Geometry: see drawing. Coordinates: mm, zero at the bounding-box minimum. A direction names the side the tool comes from. Coordinates: 2 decimals unless noted, no trailing zeros. Order: outer loops, then holes, each group sorted by start corner. A loop starts at its lowest first (then second) coordinate and runs counter-clockwise, first axis right, second up.
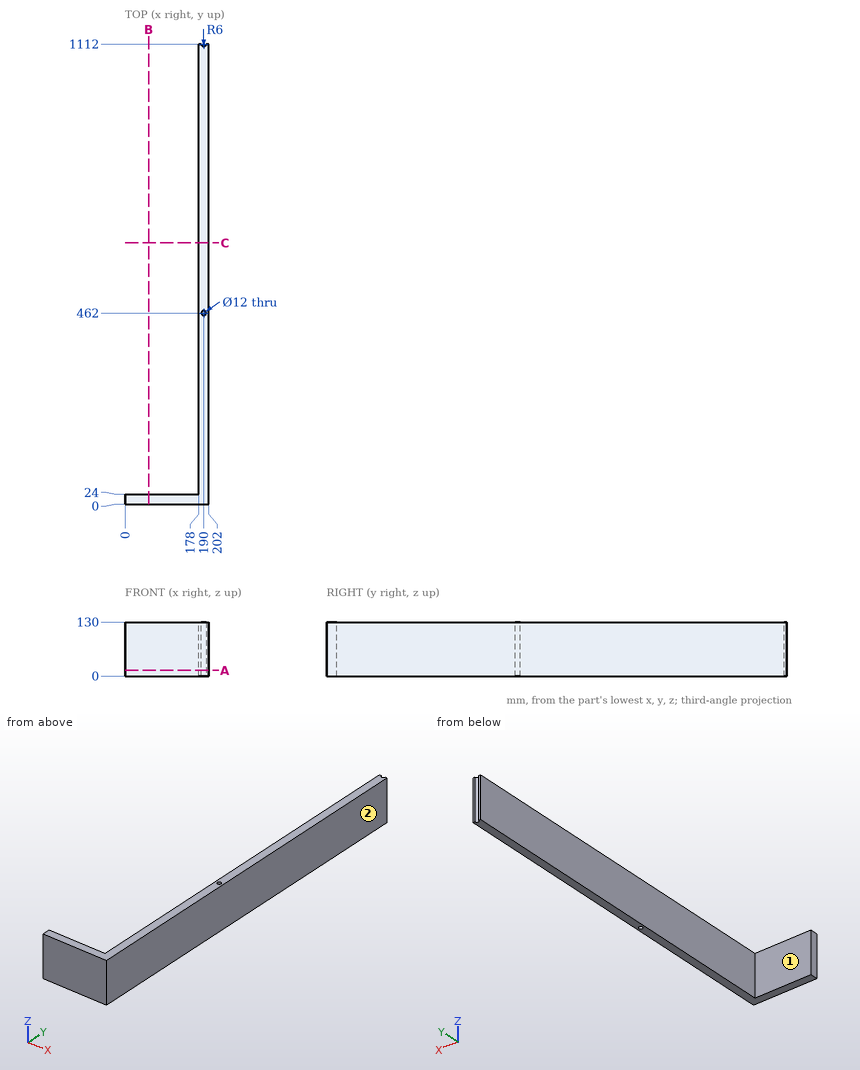
Item 1: Cut plane A-A on z = 13.5. Return loops of the section in (x, y), then the cut area to 3 significant figures.
Response values:
outline: (0, 0) - (202, 0) - (202, 1112) - (196, 1112) arc R6 cw to (184, 1112) - (178, 1112) - (178, 24) - (0, 24) - close; hole circle Ø12 at (190, 462)
area: 30,800 mm2
Item 2: Pin query (flat end, axial travel): pin 1 Ø2 at (x, z) = (142, 88) entering from +Y; pin 2 Ø8 at (y, z) = (142, 54.5) entering from -X; pin 3 Ø3 at (x, y) = (180, 131.5) entering from -Z. Return the tip coordinate at first contact, or that it passes through.
Response values:
pin 1: stops at y = 24
pin 2: stops at x = 178
pin 3: stops at z = 0
Item 3: Access query for the marked faces 1 and 2. Directions: +Z, -Z, +X, -X, +Y, -Y. A direction counts if a zero-diameter tool reaches every point of the face in a straight line with its end or side. Return the directions, or none.
Response values:
face 1: +Z, -Z, -X, +Y
face 2: +Z, -Z, +X, +Y, -Y
Item 4: Ray query, probe 1 along Y at (x, z) = (190, 37.5); probe 2 along X at (y, z) = (462, 81.5); probe 3 along Y at (x, z) = (95, 37.5). Return the intervals inside material, ascending.
Response values:
probe 1: y = 0 to 456, 468 to 1106
probe 2: x = 178 to 184, 196 to 202
probe 3: y = 0 to 24
Item 5: Cut plane C-C on y = 631.5. Return loops of the section in (x, z), then the cut area to 3 significant figures.
Response values:
outline: (178, 0) - (202, 0) - (202, 130) - (178, 130) - close
area: 3,120 mm2
Item 6: Cut plane B-B on x = 57. Return loops of the section in (y, z).
Response values:
outline: (0, 0) - (24, 0) - (24, 130) - (0, 130) - close
